```python
from build123d import *

# Parameters (mm, degrees)
F2_R     = 6.2570278464
F3_DEPTH = 25
F5_SIZE  = 1


# Not quite as in the source:
# - a fillet or chamfer that OpenCascade refuses, or shapes differently, is made with other operations: its cross-section is extruded or revolved along the edge and cut away or added


with BuildPart() as f1:
    # F0 (on Front) → F1 (revolve)
    with BuildSketch(Plane.XZ):
        Polygon((0, 11.8446564302), (0, 8.9004915208), (11.2406639382, 8.9004915208), (11.2406639382, 11.8446564302), (7.6611181721, 11.8446564302), (7.6611181721, 29.8391282558), (14.5299769938, 29.8391282558), (14.5299769938, 33.2251861691), (0, 33.2251861691), (0, 29.8391282558), (3.4043616615, 29.8391282558), (3.4043616615, 11.8446564302), align=None)
    revolve(axis=Axis((7.4493242428, 0, 0), (1, 0, 0)))

    # F2 (on face) → F3 (cut)
    with BuildSketch(Plane.YZ.offset(7.6611181721)):
        with Locations((0, 20.9185741842)):
            Circle(F2_R)
        with Locations((19.8947462895, 6.464194921)):
            Circle(F2_R)
        with Locations((12.2956294044, -16.9234820131)):
            Circle(F2_R)
        with Locations((-12.2956294044, -16.9234820131)):
            Circle(F2_R)
        with Locations((-19.8947462895, 6.464194921)):
            Circle(F2_R)
    extrude(amount=-F3_DEPTH, mode=Mode.SUBTRACT)

    # F4: fillet of radius 5 on 3 edges, made by hand

    # F4_s1 → F4_t2 (revolve, cut)
    with BuildSketch(Plane.XZ):
        with BuildLine():
            ThreePointArc((9.7976212442, 33.2251861691), (12.7071134307, 32.2914934887), (14.5299769938, 29.8391282558))
            Line((14.5299769938, 29.8391282558), (14.6246241088, 29.8714070976))
            ThreePointArc((14.6246241088, 29.8714070976), (14.6299769938, 31.5321572125), (14.6299769938, 33.2251861691))
            Line((14.6299769938, 33.2251861691), (14.5299769938, 33.3251861691))
            Line((14.5299769938, 33.3251861691), (9.7976212442, 33.3251861691))
            Line((9.7976212442, 33.3251861691), (9.7976212442, 33.2251861691))
        make_face()
    revolve(axis=Axis((14.5299769938, 0, 0), (1, 0, 0)), mode=Mode.SUBTRACT)

    # F4_s3 → F4_t4 (revolve, cut)
    with BuildSketch(Plane.XZ):
        with BuildLine():
            ThreePointArc((0, 29.8391282558), (1.8228635631, 32.2914934887), (4.7323557496, 33.2251861691))
            Line((4.7323557496, 33.2251861691), (4.7323557496, 33.3251861691))
            Line((4.7323557496, 33.3251861691), (0, 33.3251861691))
            Line((0, 33.3251861691), (-0.1, 33.2251861691))
            ThreePointArc((-0.1, 33.2251861691), (-0.1, 31.5321572125), (-0.094647115, 29.8714070976))
            Line((-0.094647115, 29.8714070976), (0, 29.8391282558))
        make_face()
    revolve(axis=Axis((0, 0, 0), (1, 0, 0)), mode=Mode.SUBTRACT)

    # F5
    f5_edges = [f1.edges().sort_by_distance(p)[0] for p in [
        (3.404362, -6.257028, 20.918574),
        (3.404362, -26.151774, 6.464195),
        (3.404362, -18.552657, -16.923482),
        (3.404362, 6.038602, -16.923482),
        (3.404362, 13.637718, 6.464195),
    ]]
    chamfer(f5_edges, length=F5_SIZE)


solid = f1.part
```
Build history of the part. All positions in model axes, mm. A direction names the side the tool comes from. Coordinates: 2 decimals unless noted, no trailing zeros. Order: outer loops, then holes, each group sorted by start corner. A loop starts at its lowest first (then second) coordinate and runs counter-clockwise, first axis right, second up. Notation, with made-up numbers: M 76,-18.75 L 99,-18.75 A30 cw 99,10.25 Z; hole C 24,43 d5. An arc over 180 degrees is marked long. One line per question, with ' | ' between items. Start each with the question number.
1. Wall check: line 1 along Z through (x, y) = (6.75, 0); line 2 along Y through (x, z) = (9, -7.5); line 3 along Z through (x, y) = (2.45, 0). Give the ranges that are in metal, low to high. Write a range as [from, to].
2. Cut at B-B (x = 1.5). Write the cut outline in (y, z).
3. Mould opens along Z. For faces 4 (the face through (0, -9, 2)), 5 (the face through (1.73, 29.13, -6.47)), 6 (the face through (7.23, -28.016, 17.862)) say: +Z half, -Z half, draft (parallel to the pull), parting line (faces both ways), or undercut.
4. Cut at A-A (y = 0). Count the separate pieces of the cut face and the enclosed holes in it, plus the area to 3 significant figures.
5. Tool access for faces 1 (the face through (6.06, -8.93, -11.65)), 2 (the face through (1.678, -3.558, 11.298)), 3 (the face through (11.14, 29.13, -6.47)): list every direction of +Z, -Z, +X, -X, +Y, -Y with a clear straight run to the whole face (end or side of a thin tool).
6. Flat gauge pins, fed straight in: P1, Ø3, axis at y = 6, z = 25.5, coming from the -X side; P2, Ø2, axis at x = 3, y = 1.5, coming from the +Z side; P3, Ø1, axis at x = 10, y = -11, coming from the +Z side. Where does each tip first touch, or does it go through?
The answers:
1) line 1: z = [-33.23, -8.9], [8.9, 14.66], [27.18, 33.23] | line 2: y = [-32.37, -28.88], [-9.17, -4.79], [4.79, 9.17], [28.88, 32.37] | line 3: z = [-32.67, -29.84], [-11.84, -8.9], [8.9, 11.84], [29.84, 32.67]
2) outline: C 0,0 d64.08; C 0,0 d23.69; hole C 0,0 d59.68; hole C 0,0 d17.8
3) face 4: draft | face 5: undercut | face 6: parting line
4) separate pieces: 3 | enclosed holes: 0 | area: 246 mm2
5) face 1: +X, -X | face 2: -X | face 3: +X
6) P1: stops at x = 3.4 | P2: stops at z = 33.14 | P3: stops at z = 31.52
